```python
from build123d import *

# Parameters (mm, degrees)
F1_DEPTH = 1111.25
F2_W     = 122.435573
F2_H     = 50.8
F2_W_2   = 93.867282
F2_W_3   = 343.160421
F2_H_2   = 127
F3_DEPTH = 25.4
F4_R     = 0.79375
F5_DEPTH = 25.4
F6_R     = 4.7625
F7_DEPTH = 25.4


with BuildPart() as f1:
    # F0 (on Top) → F1 (new body)
    with BuildSketch(Plane.XY):
        Polygon((7.890768, -9.525), (0, 9.525), (-25.4, 9.525), (-25.4, -9.525), align=None)
    extrude(amount=F1_DEPTH)

    # F2 (on Front) → F3 (cut)
    with BuildSketch(Plane.XZ):
        with Locations((22.446524, 25.4)):
            Rectangle(F2_W, F2_H)
        with Locations((2.720783, 755.65)):
            Rectangle(F2_W_2, F2_H)
        with Locations((-38.781822, 1047.75)):
            Rectangle(F2_W_3, F2_H_2)
    extrude(amount=F3_DEPTH, mode=Mode.SUBTRACT)

    # F4 (on Front) → F5 (cut)
    with BuildSketch(Plane.XZ):
        with Locations((12.7, 101.6)):
            Circle(F4_R)
        with Locations((12.7, 155.575)):
            Circle(F4_R)
        with Locations((12.7, 625.475)):
            Circle(F4_R)
        with Locations((12.7, 679.45)):
            Circle(F4_R)
        with Locations((-12.7, 625.475)):
            Circle(F4_R)
        with Locations((-12.7, 679.45)):
            Circle(F4_R)
        with Locations((-12.7, 101.6)):
            Circle(F4_R)
        with Locations((-12.7, 155.575)):
            Circle(F4_R)
    extrude(amount=-F5_DEPTH, mode=Mode.SUBTRACT)

    # F6 (on Front) → F7 (cut)
    with BuildSketch(Plane.XZ):
        with Locations((-15.875, 254)):
            Circle(F6_R)
        with Locations((-15.875, 482.6)):
            Circle(F6_R)
    extrude(amount=F7_DEPTH, mode=Mode.SUBTRACT)


solid = f1.part
```
CAD build for the part. Positions are in the model's coordinates, mm. A direction names the side the tool comes from. Give positions to 0.01 mm unless a question says otherwise; leave off trailing zeros. Order: outer loops, then holes, each group sorted by start corner. A loop starts at its lowest first (then second) coordinate and runs counter-clockwise, first axis right, second up.
(1) Flat gauge pins, fed straight in: pin 1 (9 mm diameter, centred on x = -5, z = 34.5, fed in from -Y); pin 2 (0.8 mm diameter, centred on x = -12.5, z = 101.5, fed in from +Y); pin 3 (3 mm diameter, centred on x = -8, y = -6, fed in from -Z). Where does each tip first touch, or does it go through?
(2) Mould opens along Z. For faces 1 (the flat face through (4, -0.13, 547.85)), 2 (the flat face through (-11, 0, 756)) say: released by +Z, released by -Z, zero draft, split by the parting line, or undercut.
(3) Drill centre lines: L1, parallel to Z at x = -12.7, y = 4.75; L2, parallel to Z at x = -6, y = -2; L3, parallel to Z at x = -13, y = 0.5. Where is each one in solid material? Low to high.
(4) Saw through at B-B, the plane z = 888.5. Give the cut face in (x, y) (3 decimals), then the cut area to 3 significant figures.
(5) Saw through at A-A, the plane y = -6. State how many separate pieces and enclosed holes the cut face has, then the cut area to 3 significant figures.
(6) Tool access for faces 3 (the flat face through (-11, 0, 1049)), 4 (the flat face through (-9, -9.525, 386)), 5 (the flat face through (-11, 0, 26)): list every direction of +Z, -Z, +X, -X, +Y, -Y with a clear straight run to the whole face (end or side of a thin tool).
Results found:
1. pin 1: stops at y = 0
1. pin 2: stops at y = 0
1. pin 3: stops at z = 50.8
2. face 1: zero draft
2. face 2: undercut
3. L1: z = 0 to 100.81, 102.39 to 154.78, 156.37 to 624.68, 626.27 to 678.66, 680.24 to 1111.25
3. L2: z = 50.8 to 730.25, 781.05 to 984.25
3. L3: z = 0 to 100.87, 102.33 to 154.84, 156.31 to 624.74, 626.21 to 678.72, 680.18 to 1111.25
4. outline: (-25.4, -9.525) - (7.891, -9.525) - (0, 9.525) - (-25.4, 9.525) - close
4. area: 559 mm2
5. separate pieces: 2
5. enclosed holes: 2
5. area: 28,000 mm2
6. face 3: +Z, +X, -X, -Y
6. face 4: +Z, -Z, +X, -X, -Y
6. face 5: -Z, +X, -X, -Y
